The model under review builds one solid part; all positions refer to its coordinate system, in mm. Face numbers are marked on the shaded views. A direction names the side the tool comes from. Give positions to 0.01 mm unless a question says otherwise; leave off trailing zeros. Loops run counter-clockwise (first coordinate to the right, second up) from the corner with the lowest first, then second, coordinate; pieces in that order, holes last. Notation, with made-up numbers: M -20.5,37 L 31.5,37 A28 ccw 31.5,57 Z; hole C -18,57.25 d7. An arc over 180 degrees is marked long. One line per item, written item: value. Start each with the question number.
Q1. For pin 1 (8 mm diameter, centred on x = -27, y = -3, fed in from +Z); pin 2 (2.5 mm diameter, centred on y = -17.5, z = 8, fed in from +X); pin 3 (8 mm diameter, centred on x = -28.5, z = 14.5, fed in from -Y); pin 4 (3.5 mm diameter, centred on y = 17.5, z = 14, fed in from -X), all flat-tipped, find the tip position at first contact; note any pin that passes through.
Q2. We need section D-D on x = -30.5. Write out the cut boundary in (y, z).
Q3. To check wall thickness, follow line 1 along Z through (x, y) = (-22.9, -17.5); line 2 along Y through (x, z) = (-23, 1.5); line 3 along Z through (x, y) = (-21.75, 17). State the ranges of each line that lie inside material, in increasing order. Write a range as from..to.
Q4. We need section A-A on z = 8. Write out the cut boundary in (x, y), plus the area to 3 significant figures.
Q5. We need section C-C on z = 10.75. Write out the cut boundary in (x, y).
Q6. We need section B-B on y = 0. Write out the cut boundary in (x, z).
Q7. For the marked faces 1 and 2, list the 3-axis set-ups (+Z, -Z, +X, -X, +Y, -Y) from which the entire face can be reached by the end or side of a thin tool; tool diameter is ignored.
```python
from build123d import *

# Parameters (mm, degrees)
SKETCH_1_R          = 1.5
EXTRUDE_1_DEPTH     = 17
SKETCH_3_W          = 9.079689783
SKETCH_3_H          = 45.034094638
CUT_EXTRUDE_2_DEPTH = 12
SKETCH_5_R          = 1.5
CUT_EXTRUDE_3_DEPTH = 32.503374865


with BuildPart() as part:
    # 草图1 → 凸台-拉伸1 (new body)
    with BuildSketch(Plane.XY):
        with BuildLine():
            Line((-24.691948814, 23.068360514), (-33.771638598, 1.148050297))
            ThreePointArc((-33.771638598, 1.148050297), (-34, 0), (-33.771638598, -1.148050297))
            Line((-33.771638598, -1.148050297), (-24.691948814, -23.068360514))
            ThreePointArc((-24.691948814, -23.068360514), (-21.335039251, -24.862666058), (-18.920310217, -21.920310217))
            Line((-18.920310217, -21.920310217), (-18.920310217, 21.920310217))
            ThreePointArc((-18.920310217, 21.920310217), (-21.335039251, 24.862666058), (-24.691948814, 23.068360514))
        make_face()
        with Locations((-31, 0)):
            Circle(SKETCH_1_R, mode=Mode.SUBTRACT)
        with Locations((-21.920310217, 21.920310217)):
            Circle(SKETCH_1_R, mode=Mode.SUBTRACT)
        with Locations((-21.920310217, -21.920310217)):
            Circle(SKETCH_1_R, mode=Mode.SUBTRACT)
    extrude(amount=EXTRUDE_1_DEPTH)

    # 草图3 → 切除-拉伸2 (cut)
    with BuildSketch(Plane.XY.offset(17)):
        with Locations((-29.460155109, 0)):
            Rectangle(SKETCH_3_W, SKETCH_3_H)
    extrude(amount=-CUT_EXTRUDE_2_DEPTH, mode=Mode.SUBTRACT)

    # 草图5 → 切除-拉伸3 (cut, through all)
    with BuildSketch(Plane.ZY.offset(24.920310217)):
        with Locations(Location((8, 17.5, 0), (0, 0, 270))):
            Circle(SKETCH_5_R)
        with Locations(Location((14, 17.5, 0), (0, 0, 90))):
            Circle(SKETCH_5_R)
        with Locations(Location((14, -17.5, 0), (0, 0, 270))):
            Circle(SKETCH_5_R)
        with Locations(Location((8, -17.5, 0), (0, 0, 90))):
            Circle(SKETCH_5_R)
    extrude(amount=-CUT_EXTRUDE_3_DEPTH, mode=Mode.SUBTRACT)


solid = part.part
```
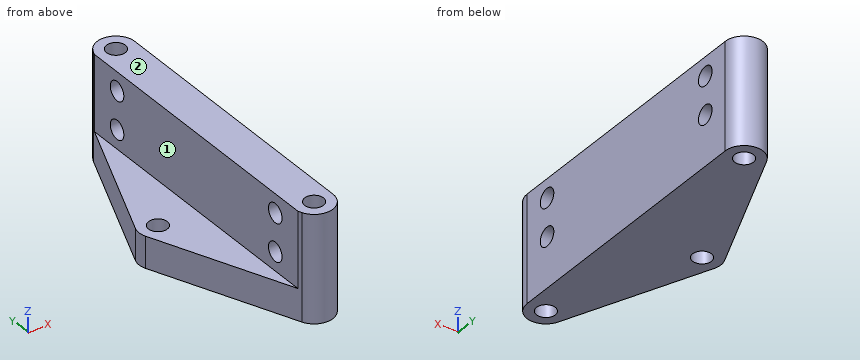
Solved:
1. pin 1: z = 17
1. pin 2: through
1. pin 3: y = -23.45
1. pin 4: x = -24.92
2. outline: M -9.05,0 L -1.41,0 L -1.41,5 L -9.05,5 Z; M 1.41,0 L 9.05,0 L 9.05,5 L 1.41,5 Z
3. line 1: 0..6.5, 9.5..12.5, 15.5..17
3. line 2: -24.72..-22.96, -20.88..20.88, 22.96..24.72
3. line 3: 0..6.59, 9.41..12.59, 15.41..17
4. outline: M -24.92,-22.52 L -24.69,-23.07 A3 ccw -18.92,-21.92 L -18.92,-19 L -24.92,-19 Z; M -24.92,-16 L -18.92,-16 L -18.92,16 L -24.92,16 Z; M -24.92,19 L -18.92,19 L -18.92,21.92 A3 ccw -24.69,23.07 L -24.92,22.52 Z; hole C -21.92,-21.92 d3; hole C -21.92,21.92 d3
4. area: 241 mm2
5. outline: M -24.92,-22.52 L -24.69,-23.07 A3 ccw -18.92,-21.92 L -18.92,21.92 A3 ccw -24.69,23.07 L -24.92,22.52 Z; hole C -21.92,-21.92 d3; hole C -21.92,21.92 d3
6. outline: M -34,0 L -32.5,0 L -32.5,5 L -34,5 Z; M -29.5,0 L -18.92,0 L -18.92,17 L -24.92,17 L -24.92,5 L -29.5,5 Z
7. face 1: +Z, -X, +Y, -Y
7. face 2: +Z, +X, -X, +Y, -Y
